```python
from build123d import *

# Parameters (mm, degrees)
BOSS_EXTRUDE1_DEPTH = 750
SKETCH1_3_W         = 1100
SKETCH1_3_H         = 600
CUT_EXTRUDE1_DEPTH  = 100
FILLET1_R           = 50.000000076
SKETCH2_W           = 47
SKETCH2_H           = 80.5
BOSS_EXTRUDE2_DEPTH = 66.215


with BuildPart() as part:
    # Sketch1 → Boss-Extrude1 (new body)
    with BuildSketch(Plane(origin=(0, 0, 0), x_dir=(1, 0, 0), z_dir=(0, 1, 0))):
        with BuildLine():
            Line((-730, 350), (730, 350))
            ThreePointArc((730, 350), (814.852813742, 314.852813742), (850, 230))
            Line((850, 230), (850, -230))
            ThreePointArc((850, -230), (814.852813742, -314.852813742), (730, -350))
            Line((730, -350), (-730, -350))
            ThreePointArc((-730, -350), (-814.852813742, -314.852813742), (-850, -230))
            Line((-850, -230), (-850, 230))
            ThreePointArc((-850, 230), (-814.852813742, 314.852813742), (-730, 350))
        make_face()
    extrude(amount=-BOSS_EXTRUDE1_DEPTH)

    # Sketch1_3 → Cut-Extrude1 (cut)
    with BuildSketch(Plane(origin=(0, 0, 0), x_dir=(1, 0, 0), z_dir=(0, 1, 0))):
        Rectangle(SKETCH1_3_W, SKETCH1_3_H)
    extrude(amount=-CUT_EXTRUDE1_DEPTH, mode=Mode.SUBTRACT)

    # Fillet1
    fillet1_edges = [part.edges().sort_by_distance(p)[0] for p in [
        (550, -50, -300),
        (550, -50, 300),
        (-550, -50, 300),
        (-550, -50, -300),
    ]]
    fillet(fillet1_edges, radius=FILLET1_R)

    # Sketch2 → Boss-Extrude2 (add)
    with BuildSketch(Plane.XZ.offset(750)):
        with Locations((-775.7, 258.95)):
            Rectangle(SKETCH2_W, SKETCH2_H)
        with Locations((775.7, 258.95)):
            Rectangle(SKETCH2_W, SKETCH2_H)
        with Locations((775.7, -258.95)):
            Rectangle(SKETCH2_W, SKETCH2_H)
        with Locations((-775.7, -258.95)):
            Rectangle(SKETCH2_W, SKETCH2_H)
    extrude(amount=BOSS_EXTRUDE2_DEPTH)


solid = part.part
```
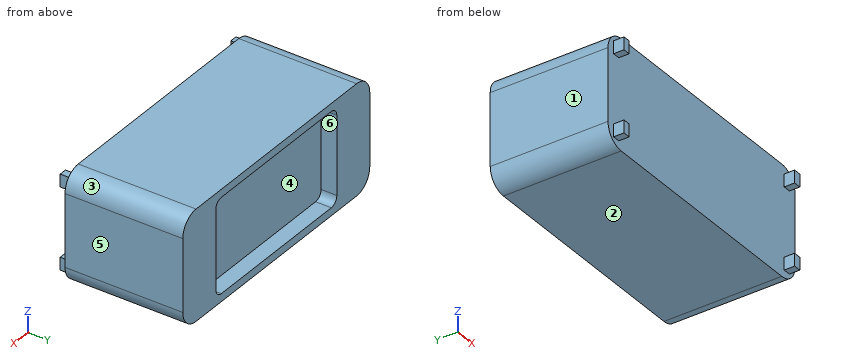
Work out the finished part from the listing and answer in its coordinate system (mm). Face numbers are marked on the shaded views. A direction names the side the tool comes from. Round coordinates to 2 decimals unless told otherwise and drop trailing zeros. Write each loop counter-clockwise with the first axis right and the second up, starting at its lowest first coordinate (ties: lowest second). Pieces come first, ordered by that corner, then holes.
1) Determine the mould class of the marked faces 1, 2, 3 and 4 for opening direction X: pulls with the +X half, pulls with the -X half, needs draft (parallel to the pull), parting line crosses it, or undercut.
2) A cutting plane is placed at B-B on x = -466.5. Determine the outline of the cut face in (y, z).
3) Flat-ended cylindrical pins translate along their axes: P1, Ø23.5, axis at x = -781.5, y = -782, coming from the +Z side; P2, Ø10, axis at x = 295.5, z = 259, coming from the +Y side; P3, Ø20, axis at y = -776, z = -264.5, coming from the -X side. Find the tip coordinate at first contact, or state that the pin passes through.
4) A cutting plane is placed at C-C on x = 657.5. Determine the outline of the cut face in (y, z), and give its area (3 significant figures).
5) A cutting plane is placed at A-A on z = 17. Determine the outline of the cut face in (x, y), and give its area (4 significant figures).
6) Consider probe 1 along Z at (x, y) = (394, -67.5); probe 2 along Y at (x, z) = (-487.5, 65.5); probe 3 along Y at (x, z) = (-590.5, 57). Determine where each line is inside the solid, lowest interval first.
7) Which of the six approach directions +Z, -Z, +X, -X, +Y, -Y give full straight-line access (tool end or side, diameter ignored) to the marked faces 5 and 6?
Entries:
1. face 1: pulls with the -X half
1. face 2: needs draft
1. face 3: pulls with the +X half
1. face 4: undercut
2. outline: (-750, -350) - (0, -350) - (0, -300) - (-100, -300) - (-100, 300) - (0, 300) - (0, 350) - (-750, 350) - close
3. P1: stops at z = 299.2
3. P2: stops at y = -100
3. P3: stops at x = -799.2
4. outline: (-750, -350) - (0, -350) - (0, 350) - (-750, 350) - close
4. area: 525,000 mm2
5. outline: (-850, -750) - (850, -750) - (850, 0) - (550, 0) - (550, -100) - (-550, -100) - (-550, 0) - (-850, 0) - close
5. area: 1,165,000 mm2
6. probe 1: z = -350 to -300, 300 to 350
6. probe 2: y = -750 to -100
6. probe 3: y = -750 to 0
7. face 5: +Z, -Z, +X, +Y, -Y
7. face 6: +Y
